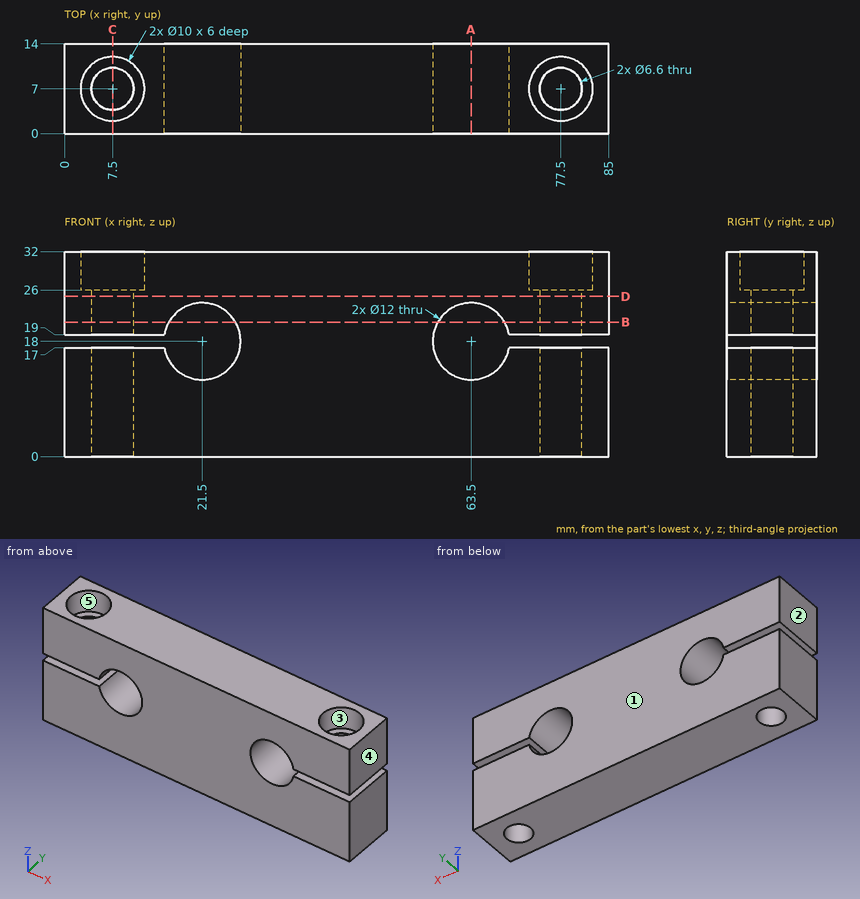
Here's the drawing with two shaded views (mm, measured from the low corner). I have some questions. A direction names the side the tool comes from. Coordinates: 2 decimals unless noted, no trailing zeros. Write each loop counter-clockwise with the first axis right and the second up, starting at its lowest first coordinate (ties: lowest second). Pieces come first, ordered by that corner, then holes. Notation, with made-up numbers: M 73.25,79 L 116.25,79 A13 ccw 116.25,86 Z; hole C 9,-31.5 d10. An arc over 180 degrees is marked long. Answer as CSV lines item,"result". Start each with the question number.
1) I want a section at C-C, the plane x = 7.5. Please give me the cut outline in (y, z).
2) I want a section at A-A, the plane x = 63.5. Please give me the cut outline in (y, z), and give its area (3 significant figures).
3) I want a section at D-D, the plane z = 25. Please give me the cut outline in (x, y).
4) For P1, Ø8, axis at x = 77.5, y = 7, coming from the +Z side; P2, Ø6, axis at x = 77.5, y = 7, coming from the +Z side, each with a flat end and sliding along its axis, tell me the tip position at first contact or that it passes through.
5) I want a section at B-B, the plane z = 21. Please give me the cut outline in (x, y).
6) We'd pull the mould along Y, two halves only. Please class the marked faces 1, 2 and 3: +Y half, -Y half, draft (parallel to the pull), parting line (faces both ways), or undercut.
7) For the marked faces 4 and 5, which set-ups out of +Z, -Z, +X, -X, +Y, -Y let a thin tool reach every point of the face, with its end or its side?
8) Please list where these lines run through material, in increasing order: line 1 (X direction, y = 7, z = 6); line 2 (Z direction, x = 21.5, y = 9.5); line 3 (X direction, y = 5.75, z = 13). Write a range as from..to.
Data:
1,outline,"M 0,0 L 3.7,0 L 3.7,17 L 0,17 Z; M 0,19 L 3.7,19 L 3.7,26 L 2,26 L 2,32 L 0,32 Z; M 10.3,0 L 14,0 L 14,17 L 10.3,17 Z; M 10.3,19 L 14,19 L 14,32 L 12,32 L 12,26 L 10.3,26 Z"
2,outline,"M 0,0 L 14,0 L 14,12 L 0,12 Z; M 0,24 L 14,24 L 14,32 L 0,32 Z"
2,area,"280 mm^2"
3,outline,"M 0,0 L 85,0 L 85,14 L 0,14 Z; hole C 7.5,7 d6.6; hole C 77.5,7 d6.6"
4,P1,"stops at z = 26"
4,P2,"passes through"
5,outline,"M 0,0 L 16.3,0 L 16.3,14 L 0,14 Z; M 26.7,0 L 58.3,0 L 58.3,14 L 26.7,14 Z; M 68.7,0 L 85,0 L 85,14 L 68.7,14 Z; hole C 7.5,7 d6.6; hole C 77.5,7 d6.6"
6,face 1,"+Y half"
6,face 2,"draft"
6,face 3,"undercut"
7,face 4,"+Z, -Z, +X, +Y, -Y"
7,face 5,"+Z"
8,line 1,"x = 0..4.2, 10.8..74.2, 80.8..85"
8,line 2,"z = 0..12, 24..32"
8,line 3,"x = 0..4.45, 10.55..18.18, 24.82..60.18, 66.82..74.45, 80.55..85"
